Geometry check sheet. Reference: drawing and pictorial views, mm from the part's lowest x, y, z. A direction names the side the tool comes from. Coordinates: 2 decimals unless noted, no trailing zeros. Loops run counter-clockwise (first coordinate to the right, second up) from the corner with the lowest first, then second, coordinate; pieces in that order, holes last. Notation, with made-up numbers: (58, 1) -> (65, 1) arc R37 ccw to (65, 40) -> close; hole circle Ø9 at (-24, -21). An arc over 180 degrees is marked (long way). Use one line per item in the form item = value.
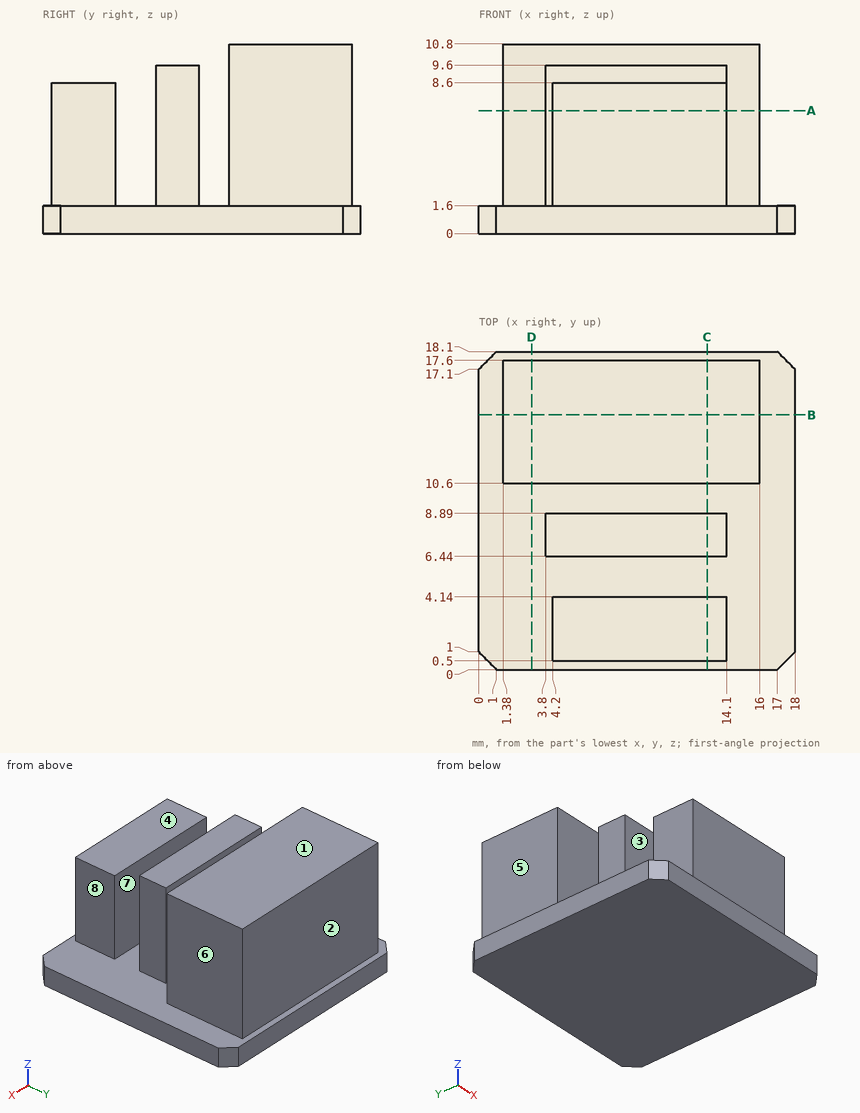
(1) Mould release check, pull along Y, two halves, no side actions. Record for the marked faces 1, 2 and 3: +Y half, -Y half, draft (parallel to the pull), parting line (faces both ways), or undercut.
Established:
face_1 = draft
face_2 = +Y half
face_3 = undercut
(2) Go/stop test with flat-tipped pins: P1, Ø1.8, axis at x = 11, y = 2, coming from the +Z side; P2, Ø1.5, axis at x = 11, z = 9, coming from the +Y side; P3, Ø5, axis at x = 5, z = 6.5, coming from the -Y side. Record where each tip stops, or that it passes through.
Established:
P1 = 8.6
P2 = 17.6
P3 = 0.5
(3) Section check C-C, the plane x = 13. Record the boundary of the cut face in (y, z), plus the area to 3 significant figures.
Established:
outline = (0, 0) -> (18.1, 0) -> (18.1, 1.6) -> (17.6, 1.6) -> (17.6, 10.8) -> (10.6, 10.8) -> (10.6, 1.6) -> (8.89, 1.6) -> (8.89, 9.6) -> (6.44, 9.6) -> (6.44, 1.6) -> (4.14, 1.6) -> (4.14, 8.6) -> (0.5, 8.6) -> (0.5, 1.6) -> (0, 1.6) -> close
area = 138 mm²
(4) Tool access check on the marked faces 4, 5, 6, 7 and 8. Record the directions out of +Z, -Z, +X, -X, +Y, -Y that give a thin tool (end or side, any length) a straight path to the whole face; none if there is none.
Established:
face_4 = +Z, +X, -X, -Y
face_5 = +Z, -X, +Y, -Y
face_6 = +Z, +X, +Y, -Y
face_7 = +Z, +X, -X
face_8 = +Z, +X, -Y
(5) Section check B-B, the plane y = 14.5. Record the boundary of the cut face in (x, z).
Established:
outline = (0, 0) -> (18, 0) -> (18, 1.6) -> (16, 1.6) -> (16, 10.8) -> (1.38, 10.8) -> (1.38, 1.6) -> (0, 1.6) -> close
(6) Section check A-A, the plane z = 7. Record the boundary of the cut face in (x, y), plus the area to 3 significant figures.
Established:
outline = (1.38, 10.6) -> (16, 10.6) -> (16, 17.6) -> (1.38, 17.6) -> close; (3.8, 6.44) -> (14.1, 6.44) -> (14.1, 8.89) -> (3.8, 8.89) -> close; (4.2, 0.5) -> (14.1, 0.5) -> (14.1, 4.14) -> (4.2, 4.14) -> close
area = 164 mm²
(7) Scan lines: line 1 along Y through (x, z) = (10.5, 8.25); line 2 along Y through (x, z) = (4, 6.5); line 3 along Y through (x, z) = (4.25, 10.25). Record each from-to range of solid material in increasing order.
Established:
line_1 = 0.5 to 4.14, 6.44 to 8.89, 10.6 to 17.6
line_2 = 6.44 to 8.89, 10.6 to 17.6
line_3 = 10.6 to 17.6
(8) Section check D-D, the plane x = 3. Record the boundary of the cut face in (y, z).
Established:
outline = (0, 0) -> (18.1, 0) -> (18.1, 1.6) -> (17.6, 1.6) -> (17.6, 10.8) -> (10.6, 10.8) -> (10.6, 1.6) -> (0, 1.6) -> close
